```python
from build123d import *

# Parameters (mm, degrees)
F0_W     = 13
F0_H     = 12.5
F2_R     = 12.5
F2_W     = 4
F2_H     = 6
F3_DEPTH = 3
F4_W     = 7.990635
F4_H     = 2.5
F8_R     = 1


with BuildPart() as f1:
    # F0 (on Front) → F1 (revolve)
    with BuildSketch(Plane.XZ):
        with Locations((6.5, 6.25)):
            Rectangle(F0_W, F0_H)
    revolve(axis=Axis((9.685505, 0, 0), (1, 0, 0)))

    # F2 (on face) → F3 (cut)
    with BuildSketch(Plane.YZ.offset(13)):
        Circle(F2_R)
        with Locations((0, -6.5)):
            Rectangle(F2_W, F2_H, mode=Mode.SUBTRACT)
        with Locations((0, 6.5)):
            Rectangle(F2_W, F2_H, mode=Mode.SUBTRACT)
    extrude(amount=-F3_DEPTH, mode=Mode.SUBTRACT)

    # F4 (on Front) → F5 (revolve, cut)
    with BuildSketch(Plane.XZ):
        with Locations((8.995317, 1.25)):
            Rectangle(F4_W, F4_H)
    revolve(axis=Axis((7.811431, 0, 0), (1, 0, 0)), mode=Mode.SUBTRACT)

    # F6 (on Front) → F7 (revolve, cut)
    with BuildSketch(Plane.XZ):
        Polygon((0, 3.55), (0, 0), (6.232518, 0), (6.232518, 1.75), (1.8, 1.75), align=None)
    revolve(axis=Axis((5.52431, 0, 0), (1, 0, 0)), mode=Mode.SUBTRACT)

    # F8
    f8_edges = [f1.edges().sort_by_distance(p)[0] for p in [
        (10, 0, -12.5),
        (0, 0, -12.5),
    ]]
    fillet(f8_edges, radius=F8_R)


solid = f1.part
```
Geometry check sheet. Reference: the model listing, model coordinates, mm. A direction names the side the tool comes from. Coordinates: 2 decimals unless noted, no trailing zeros. Order: outer loops, then holes, each group sorted by start corner. A loop starts at its lowest first (then second) coordinate and runs counter-clockwise, first axis right, second up.
Item 1: Section check C-C (y = 0). Enter the section's corners in (x, z).
Item 2: Section check A-A (z = 0). Enter the section's corners in (x, y).
Item 3: Scan lines: line 1 along Z through (x, y) = (2.8, 0); line 2 along Z through (x, y) = (8.35, 0). Record each from-to range of solid material in increasing order.
Item 4: Depth check by flat-ended pin: pin 1 (4 mm diameter, centred on y = 0.5, z = 1, fed in from +X); pin 2 (6 mm diameter, centred on y = -4, z = -4.5, fed in from +X); pin 3 (0.9 mm diameter, centred on x = 12, y = 0.5, fed in from -Z); pin 4 (0.9 mm diameter, centred on x = 12, y = 0, fed in from +Z). Enter the tip coordinate at first touch or a pass-through.
Item 5: Section check B-B (x = 12). Enter the section's corners in (y, z), plus the area to 3 significant figures.
Item 6: Section check D-D (x = 6.75). Enter the section's corners in (y, z).
Item 7: Mould release check, pull along Y, two halves, no side actions. Record for faces 6 (the flat face through (5, -2, -1)), 7 (the flat face through (12, 0, -3.5)), 8 (the flat face through (12, 2, 6)), 9 (the conical face through (1.687, 1.818, -0.404)): released by +Y, released by -Y, zero draft, split by the parting line, or undercut.
Item 8: Tool access check on faces 1 (the cylindrical face through (7.53, 2.44, -0.54)), 2 (the flat face through (12, 0, 9.5)), 3 (the flat face through (12, 0, -9.5)), 4 (the flat face through (12, -2, -7)), 5 (the flat face through (12, 0, 3.5)). Record the directions out of +Z, -Z, +X, -X, +Y, -Y that give a thin tool (end or side, any length) a straight path to the whole face; none if there is none.
Check sheet entries:
1. outline: (0, -11.5) arc R1 ccw to (1, -12.5) - (9, -12.5) arc R1 ccw to (10, -11.5) - (10, -9.5) - (13, -9.5) - (13, -3.5) - (10, -3.5) - (10, -2.5) - (5, -2.5) - (5, -1.75) - (1.8, -1.75) - (0, -3.55) - close; (0, 3.55) - (1.8, 1.75) - (5, 1.75) - (5, 2.5) - (10, 2.5) - (10, 3.5) - (13, 3.5) - (13, 9.5) - (10, 9.5) - (10, 11.5) arc R1 ccw to (9, 12.5) - (1, 12.5) arc R1 ccw to (0, 11.5) - close
2. outline: (0, -11.5) arc R1 ccw to (1, -12.5) - (9, -12.5) arc R1 ccw to (10, -11.5) - (10, -2.5) - (5, -2.5) - (5, -1.75) - (1.8, -1.75) - (0, -3.55) - close; (0, 3.55) - (1.8, 1.75) - (5, 1.75) - (5, 2.5) - (10, 2.5) - (10, 11.5) arc R1 ccw to (9, 12.5) - (1, 12.5) arc R1 ccw to (0, 11.5) - close
3. line 1: z = -12.5 to -1.75, 1.75 to 12.5
3. line 2: z = -12.5 to -2.5, 2.5 to 12.5
4. pin 1: stops at x = 10
4. pin 2: stops at x = 13
4. pin 3: stops at z = -9.5
4. pin 4: stops at z = 9.5
5. outline: (-2, -9.5) - (2, -9.5) - (2, -3.5) - (-2, -3.5) - close; (-2, 3.5) - (2, 3.5) - (2, 9.5) - (-2, 9.5) - close
5. area: 48.0 mm2
6. outline: circle Ø25 at (0, 0); hole circle Ø5 at (0, 0)
7. face 6: undercut
7. face 7: zero draft
7. face 8: released by +Y
7. face 9: undercut
8. face 1: +X
8. face 2: +Z, +X, +Y, -Y
8. face 3: -Z, +X, +Y, -Y
8. face 4: +Z, -Z, +X, -Y
8. face 5: +X, +Y, -Y
